```python
from build123d import *

# Parameters (mm, degrees)
ESQUISSE1_R        = 6.5
ESQUISSE1_R_2      = 1.5
BOSS_EXTRU_1_DEPTH = 5
ESQUISSE3_W        = 0.3
ESQUISSE3_H        = 0.3


with BuildPart() as part:
    # Esquisse1 → Boss.-Extru.1 (new body)
    with BuildSketch(Plane.XY):
        Circle(ESQUISSE1_R)
        Circle(ESQUISSE1_R_2, mode=Mode.SUBTRACT)
    extrude(amount=BOSS_EXTRU_1_DEPTH)

    # Esquisse3 → Enlèvement de matière-Révolution1 (revolve, cut)
    with BuildSketch(Plane(origin=(0, 0, 0), x_dir=(0, 0, -1), z_dir=(1, 0, 0))):
        with Locations((-4.85, 2.65)):
            Rectangle(ESQUISSE3_W, ESQUISSE3_H)
        with Locations((-0.15, 2.65)):
            Rectangle(ESQUISSE3_W, ESQUISSE3_H)
        with Locations((-4.85, 5.15)):
            Rectangle(ESQUISSE3_W, ESQUISSE3_H)
        with Locations((-0.15, 5.15)):
            Rectangle(ESQUISSE3_W, ESQUISSE3_H)
    revolve(axis=Axis((0, 0, 5.25), (0, 0, -1)), mode=Mode.SUBTRACT)


solid = part.part
```
Geometry check sheet. Reference: the model listing, model coordinates, mm. A direction names the side the tool comes from. Round coordinates to 2 decimals unless told otherwise and drop trailing zeros. Write each loop counter-clockwise with the first axis right and the second up, starting at its lowest first coordinate (ties: lowest second). Pieces come first, ordered by that corner, then holes. Notation, with made-up numbers: (38.25, 20.25) -> (88.25, 20.25) arc R25 cw to (88.25, 48.25) -> close; hole circle Ø4 at (44.5, -20). An arc over 180 degrees is marked (long way). Put each result on its own line as item: value.
1) Cross-section at B-B, the plane y = 4.5. Enter the section's corners in (x, z).
Recorded:
outline: (-4.69, 0) -> (-2.8, 0) -> (-2.8, 0.3) -> (-2.18, 0.3) -> (-2.18, 0) -> (2.18, 0) -> (2.18, 0.3) -> (2.8, 0.3) -> (2.8, 0) -> (4.69, 0) -> (4.69, 5) -> (2.8, 5) -> (2.8, 4.7) -> (2.18, 4.7) -> (2.18, 5) -> (-2.18, 5) -> (-2.18, 4.7) -> (-2.8, 4.7) -> (-2.8, 5) -> (-4.69, 5) -> close
2) Cross-section at A-A, the plane z = 1.25. Enter the section's corners in (x, y).
Recorded:
outline: circle Ø13 at (0, 0); hole circle Ø3 at (0, 0)
3) Cross-section at C-C, the plane x = 4.75. Enter the section's corners in (y, z).
Recorded:
outline: (-4.44, 0) -> (-2.35, 0) -> (-2.35, 0.3) -> (-1.56, 0.3) -> (-1.56, 0) -> (1.56, 0) -> (1.56, 0.3) -> (2.35, 0.3) -> (2.35, 0) -> (4.44, 0) -> (4.44, 5) -> (2.35, 5) -> (2.35, 4.7) -> (1.56, 4.7) -> (1.56, 5) -> (-1.56, 5) -> (-1.56, 4.7) -> (-2.35, 4.7) -> (-2.35, 5) -> (-4.44, 5) -> close
4) Release check for a two-part mould opening along X. For faces 3 (the face through (-2.44, -0.54, 4.85)), 4 (the face through (0, -2, 5)), 5 (the face through (-5.158, -3.955, 2.465)) record: pulls with the +X half, pulls with the -X half, needs draft (parallel to the pull), parting line crosses it, or undercut.
Recorded:
face 3: undercut
face 4: needs draft
face 5: parting line crosses it
5) Depth check by flat-ended pin: P1, Ø2.5, axis at x = 0, y = 0, coming from the +Z side. Enter the tip coordinate at first touch or a pass-through.
Recorded:
P1: passes through
6) Access from +Z, -Z, +X, -X, +Y, -Y to the whole of each face (thin tool, end or side, straight path). Record for faces 1 (the face through (2.2, -2.2, 5)), 2 (the face through (0.84, 2.67, 4.85)).
Recorded:
face 1: +Z, +X, -X, +Y, -Y
face 2: +Z
7) Thickness scan on probe 1 along Y at (x, z) = (0, 1.65); probe 2 along X at (y, z) = (2, 4.8); probe 3 along Y at (x, z) = (-1.25, 3.1). Record the ranges inside material, lowest first. Write a range as from..to.
Recorded:
probe 1: y = -6.5..-1.5, 1.5..6.5
probe 2: x = -6.18..-4.91, -4.58..-1.96, -1.5..1.5, 1.96..4.58, 4.91..6.18
probe 3: y = -6.38..-0.83, 0.83..6.38
